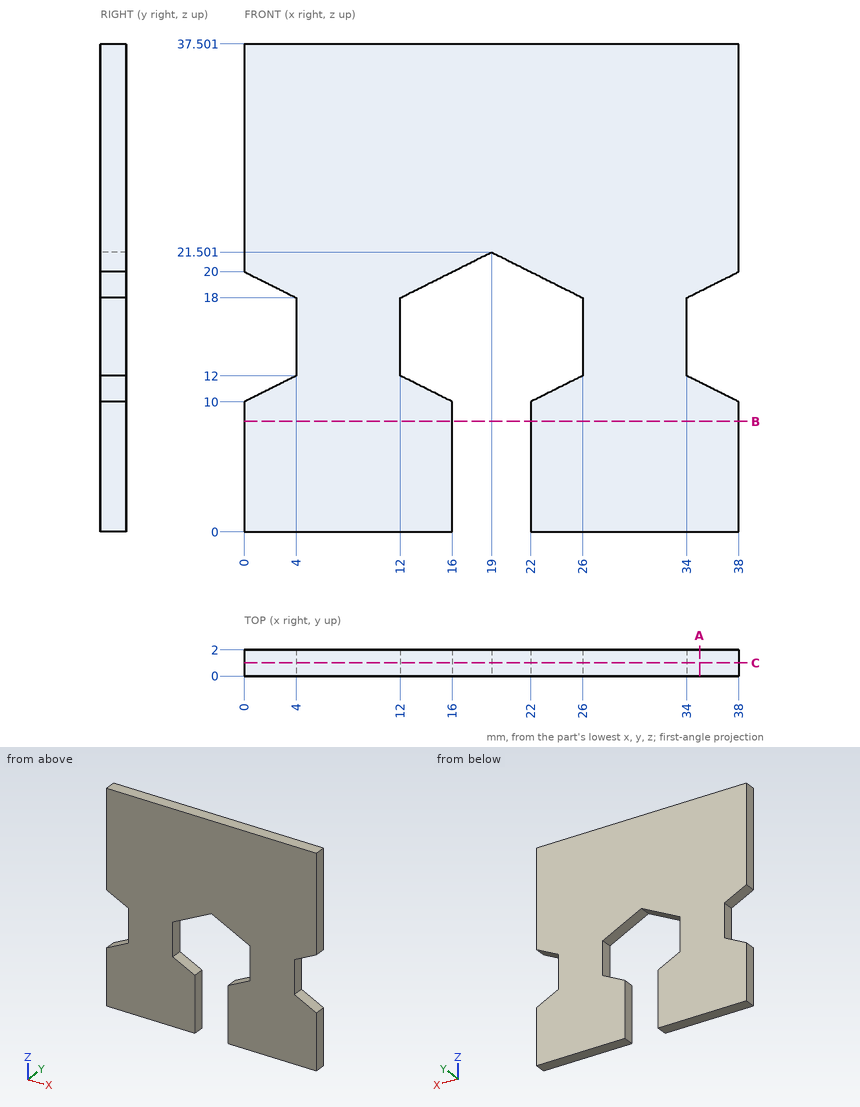
Geometry: see drawing. Coordinates: mm, zero at the bounding-box minimum. Round coordinates to 2 decimals unless told otherwise and drop trailing zeros. Loops run counter-clockwise (first coordinate to the right, second up) from the corner with the lowest first, then second, coordinate; pieces in that order, holes last. Notation, with made-up numbers: (39, 61) -> (67, 61) arc R23 ccw to (67, 99) -> close; hole circle Ø4 at (44, 22). An arc over 180 degrees is marked (long way). Write each question's results on one line, items separated by ' | '.
Item 1: Pin query (flat end, axial travel): pin 1 Ø1 at (y, z) = (1.5, 15) entering from -X. Return the tip coordinate at first contact, or that it passes through.
Answers below:
pin 1: stops at x = 4
Item 2: Cut plane C-C on y = 1. Return the cut outline in (x, z).
Answers below:
outline: (0, 0) -> (16, 0) -> (16, 10) -> (12, 12) -> (12, 18) -> (19, 21.5) -> (26, 18) -> (26, 12) -> (22, 10) -> (22, 0) -> (38, 0) -> (38, 10) -> (34, 12) -> (34, 18) -> (38, 20) -> (38, 37.5) -> (0, 37.5) -> (0, 20) -> (4, 18) -> (4, 12) -> (0, 10) -> close
Item 3: Cut plane A-A on x = 35. Return the cut outline in (y, z), and give its area (3 significant figures).
Answers below:
outline: (0, 0) -> (2, 0) -> (2, 11.5) -> (0, 11.5) -> close; (0, 18.5) -> (2, 18.5) -> (2, 37.5) -> (0, 37.5) -> close | area: 61.0 mm²
Item 4: Cut plane B-B on z = 8.5. Return the cut outline in (x, y).
Answers below:
outline: (0, 0) -> (16, 0) -> (16, 2) -> (0, 2) -> close; (22, 0) -> (38, 0) -> (38, 2) -> (22, 2) -> close
Item 5: Line query: probe 1 along X at (y, z) = (1.3, 4.5); probe 2 along Z at (x, y) = (25, 0.5); probe 3 along Z at (x, y) = (25.5, 0.3). Output: solid intervals per line, ascending. Write a range as [from, to].
Answers below:
probe 1: x = [0, 16], [22, 38] | probe 2: z = [0, 11.5], [18.5, 37.5] | probe 3: z = [0, 11.75], [18.25, 37.5]
